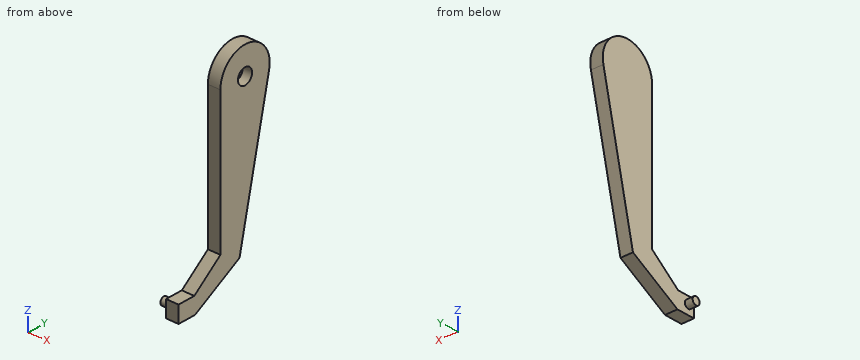
from build123d import *

# Parameters (mm, degrees)
BOSS_EXTRUDE3_DEPTH = 80
SKETCH6_R           = 50
CUT_EXTRUDE2_DEPTH  = 60
SKETCH7_R           = 25
BOSS_EXTRUDE4_DEPTH = 50


with BuildPart() as part:
    # Sketch4 → Boss-Extrude3 (new body)
    with BuildSketch(Plane(origin=(0, 0, 0), x_dir=(0, 0, -1), z_dir=(1, 0, 0))):
        with BuildLine():
            Line((1320.898617495, 319.519232733), (2260.627548778, 109.558564747))
            Line((2260.627548778, 109.558564747), (2438.924606228, -206.480811367))
            Line((2438.924606228, -206.480811367), (2438.924606228, -323.730177318))
            Line((2438.924606228, -323.730177318), (2332.658891416, -323.730177318))
            Line((2332.658891416, -323.730177318), (2332.658891416, -211.630732545))
            Line((2332.658891416, -211.630732545), (2186.534815531, -26.269822682))
            Line((2186.534815531, -26.269822682), (1282.739758098, -26.269822682))
            ThreePointArc((1282.739758098, -26.269822682), (1108.795679875, 167.925428064), (1320.898617495, 319.519232733))
        make_face()
    extrude(amount=BOSS_EXTRUDE3_DEPTH)

    # Sketch6 → Cut-Extrude2 (cut)
    with BuildSketch(Plane(origin=(80, 0, 0), x_dir=(0, 0, -1), z_dir=(1, 0, 0))):
        with Locations((1282.739758098, 148.730177318)):
            Circle(SKETCH6_R)
    extrude(amount=-CUT_EXTRUDE2_DEPTH, mode=Mode.SUBTRACT)

    # Sketch7 → Boss-Extrude4 (add)
    with BuildSketch(Plane.ZY):
        with Locations(Location((-2378.924606228, -283.730177318, 0), (0, 0, 180))):
            Circle(SKETCH7_R)
    extrude(amount=BOSS_EXTRUDE4_DEPTH)


solid = part.part
Check sheet for the modelled part. Datum: model origin and axes. Units: mm. Give positions to 0.01 mm unless a question says otherwise; leave off trailing zeros. Loops run counter-clockwise (first coordinate to the right, second up) from the corner with the lowest first, then second, coordinate; pieces in that order, holes last. Notation, with made-up numbers: M -0.5,67.5 L 16.5,67.5 A25 cw 16.5,100.5 Z; hole C 46,31 d2. An arc over 180 degrees is marked long. Return JSON: item names as keys, results as strings. Group by question number.
1. Thickness scan on L1, parallel to X at y = 252, z = -1176; L2, parallel to Y at x = 7.5, z = -1319.5; L3, parallel to Y at x = 71.5, z = -1319. Record the ranges inside material, lowest first.
2. Cross-section at A-A on x = 60.5. Record the boundary of the cut face in (y, z), plus the area to 3 significant figures.
3. Cross-section at B-B on y = 224. Record the boundary of the cut face in (x, z), plus the area to 3 significant figures.
4. Go/stop test with flat-tipped pins: pin 1 (8 mm diameter, centred on x = 48.5, z = -1511, fed in from +Y); pin 2 (8 mm diameter, centred on x = 24.5, z = -2193, fed in from +Y); pin 3 (3 mm diameter, centred on x = 3.5, z = -1584.5, fed in from +Y). Record where each tip stops, or that it passes through.
5. Cross-section at C-C on z = -1912.5. Record the boundary of the cut face in (x, y).
Return value:
{
 "1": {"L1": "0 to 80", "L2": "-26.27 to 319.83", "L3": "-26.27 to 114.3, 183.16 to 319.93"},
 "2": {"outline": "M -323.73,-2438.92 L -206.48,-2438.92 L 109.56,-2260.63 L 319.52,-1320.9 A175 ccw long -26.27,-1282.74 L -26.27,-2186.53 L -211.63,-2332.66 L -323.73,-2332.66 Z; hole C 148.73,-1282.74 d100", "area": "321,000 mm^2"},
 "3": {"outline": "M 0,-1748.42 L 80,-1748.42 L 80,-1124.75 L 0,-1124.75 Z", "area": "49,900 mm^2"},
 "4": {"pin 1": "y = 277.94", "pin 2": "y = 125.56", "pin 3": "y = 260.96"},
 "5": {"outline": "M 0,-26.27 L 80,-26.27 L 80,187.34 L 0,187.34 Z"}
}
